from build123d import *

# Parameters (mm, degrees)
SKETCH_R  = 1.5
PAD_DEPTH = 1.6


with BuildPart() as part:
    # Sketch → Pad (new body)
    with BuildSketch(Plane.XY):
        with BuildLine():
            ThreePointArc((59, 0), (42.5, 6.5), (26, 0))
            Line((26, 0), (26, 53))
            ThreePointArc((26, 53), (42.5, 46.5), (59, 53))
            ThreePointArc((65.5, 53), (62.25, 53.921337), (59, 53))
            ThreePointArc((65.5, 53), (75.535332, 48.697616), (86.38794, 47.497906))
            ThreePointArc((89.147059, 43.088235), (89.043198, 46.091272), (86.38794, 47.497906))
            ThreePointArc((89.147059, 43.088235), (85, 26.5), (89.147059, 9.911765))
            ThreePointArc((86.38794, 5.502094), (89.043198, 6.908728), (89.147059, 9.911765))
            ThreePointArc((86.38794, 5.502094), (75.535332, 4.302384), (65.5, 0))
            ThreePointArc((59, 0), (62.25, -0.921337), (65.5, 0))
        make_face()
        with Locations((86.5, 44.5)):
            Circle(SKETCH_R, mode=Mode.SUBTRACT)
        with Locations((86.5, 8.5)):
            Circle(SKETCH_R, mode=Mode.SUBTRACT)
    extrude(amount=PAD_DEPTH)


solid = part.part
Source: CAD feature listing. Evaluate the final solid. Frame: model axes, mm. Give positions to 0.01 mm unless a question says otherwise; leave off trailing zeros. Write each loop counter-clockwise with the first axis right and the second up, starting at its lowest first coordinate (ties: lowest second). Pieces come first, ordered by that corner, then holes. Notation, with made-up numbers: (39, 74) -> (77, 74) arc R20 cw to (77, 98) -> close; hole circle Ø6 at (59, 14). An arc over 180 degrees is marked (long way). Return JSON: item names as keys, results as strings. Group by question number.
1. Section D-D, the plane y = 16.5. Output: boundary loops of the cut face in (x, z), then the cut area to 3 significant figures.
2. Mould query, pull axis X, two halves, no side actions, for faces 1 (the face through (58, 27, 0)), 2 (the face through (87.886, 7.925, 0.789)), 3 (the face through (85, 26.7, 0.8)). Classes: +X half, -X half, draft (parallel to the pull), parting line (faces both ways), or undercut.
3. Section C-C, the plane x = 33. Output: boundary loops of the cut face in (y, z).
4. Section B-B, the plane z = 0.5. Output: boundary loops of the cut face in (x, y).
5. Material intervals for line 1 (X direction, y = 2.5, z = 0.85); line 2 (X direction, y = 29.5, z = 0.8); line 3 (X direction, y = 36, z = 0.9), sorted ascending. Write a range as from..to.
6. Pin query (flat end, axial travel): pin 1 Ø5 at (x, y) = (86.5, 44.5) entering from -Z. Return the tip coordinate at first contact, or that it passes through.
7. Section A-A, the plane y = 44.5. Output: boundary loops of the cut face in (x, z).
Determined:
{
 "1": {"outline": "(26, 0) -> (86.45, 0) -> (86.45, 1.6) -> (26, 1.6) -> close", "area": "96.7 mm2"},
 "2": {"face 1": "draft", "face 2": "undercut", "face 3": "+X half"},
 "3": {"outline": "(4.56, 0) -> (48.44, 0) -> (48.44, 1.6) -> (4.56, 1.6) -> close"},
 "4": {"outline": "(26, 0) arc R24.19 cw to (59, 0) arc R6.19 ccw to (65.5, 0) arc R37.16 cw to (86.39, 5.5) arc R3 ccw to (89.15, 9.91) arc R35.25 cw to (89.15, 43.09) arc R3 ccw to (86.39, 47.5) arc R37.16 cw to (65.5, 53) arc R6.19 ccw to (59, 53) arc R24.19 cw to (26, 53) -> close; hole circle Ø3 at (86.5, 8.5); hole circle Ø3 at (86.5, 44.5)"},
 "5": {"line 1": "x = 26..29.18, 55.82..70.31", "line 2": "x = 26..85.13", "line 3": "x = 26..86.3"},
 "6": {"pin 1": "stops at z = 0"},
 "7": {"outline": "(26, 0) -> (85, 0) -> (85, 1.6) -> (26, 1.6) -> close; (88, 0) -> (89.5, 0) -> (89.5, 1.6) -> (88, 1.6) -> close"}
}
